The listing builds one solid part. Answer for the finished solid, in the listing's coordinates (mm). Face numbers are marked on the shaded views. A direction names the side the tool comes from. Round coordinates to 2 decimals unless told otherwise and drop trailing zeros. Write each loop counter-clockwise with the first axis right and the second up, starting at its lowest first coordinate (ties: lowest second). Pieces come first, ordered by that corner, then holes. Notation, with made-up numbers: M -33,26.5 L 10,26.5 A21 cw 10,35.5 Z; hole C 34,77 d1. An arc over 180 degrees is marked long. Write each question's results on one line, items separated by ' | '.
from build123d import *

# Parameters (mm, degrees)
CROQUIS1_W              = 50
CROQUIS1_H              = 100
SALIENTE_EXTRUIR1_DEPTH = 6
CROQUIS2_W              = 50
CROQUIS2_H              = 6
SALIENTE_EXTRUIR2_DEPTH = 276
CROQUIS3_R              = 13
CORTAR_EXTRUIR1_DEPTH   = 6
REDONDEO1_R             = 20


with BuildPart() as part:
    # Croquis1 → Saliente-Extruir1 (new body)
    with BuildSketch(Plane(origin=(0, 0, 0), x_dir=(1, 0, 0), z_dir=(0, 1, 0))):
        Rectangle(CROQUIS1_W, CROQUIS1_H)
    extrude(amount=SALIENTE_EXTRUIR1_DEPTH)

    # Croquis2 → Saliente-Extruir2 (add)
    with BuildSketch(Plane.XZ):
        with Locations((0, 53)):
            Rectangle(CROQUIS2_W, CROQUIS2_H)
    extrude(amount=-SALIENTE_EXTRUIR2_DEPTH)

    # Croquis3 → Cortar-Extruir1 (cut)
    with BuildSketch(Plane.XY.offset(56)):
        with Locations((0, 246)):
            Circle(CROQUIS3_R)
    extrude(amount=-CORTAR_EXTRUIR1_DEPTH, mode=Mode.SUBTRACT)

    # Redondeo1
    redondeo1_edges = [part.edges().sort_by_distance(p)[0] for p in [
        (25, 276, 53),
        (-25, 276, 53),
    ]]
    fillet(redondeo1_edges, radius=REDONDEO1_R)


solid = part.part
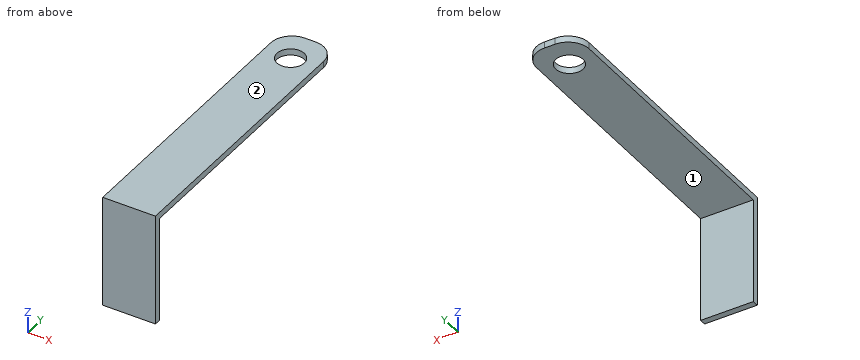
1) Find the intervals of material crossed by line 1 (Y direction, x = 0, z = 51.4); line 2 (Z direction, x = 11, y = 161); line 3 (Y direction, x = -17.5, z = -36), in increasing order.
Return value:
line 1: 0 to 233, 259 to 276 | line 2: 50 to 56 | line 3: 0 to 6
2) Section C-C (z = 11) is taken. Determine the outline of the cut face in (x, y).
Return value:
outline: M -25,0 L 25,0 L 25,6 L -25,6 Z
3) A tool of negligible diameter and unlimited length cuts with its end or side. For the marked faces 1 and 2, from which of +Z, -Z, +X, -X, +Y, -Y can it reach the whole face along a straight path? Write none if from no direction.
Return value:
face 1: -Z, +X, -X, +Y | face 2: +Z, +X, -X, +Y, -Y
4) Each of these flat-tipped pins is pushed along its axis until it touches: pin 1 (10 mm diameter, centred on x = -18.5, z = 31, fed in from +Y); pin 2 (25 mm diameter, centred on x = 8.5, y = 131, fed in from -Z). Where does it stop, or does it pass through?
Return value:
pin 1: y = 6 | pin 2: z = 50
5) Section A-A (y = 246) is taken. Determine the outline of the cut face in (x, z), then the cut area to 3 significant figures.
Return value:
outline: M -25,50 L -13,50 L -13,56 L -25,56 Z; M 13,50 L 25,50 L 25,56 L 13,56 Z | area: 144 mm²
6) Section B-B (x = 0) is taken. Determine the outline of the cut face in (y, z), then the cut area to 3 significant figures.
Return value:
outline: M 0,-50 L 6,-50 L 6,50 L 233,50 L 233,56 L 0,56 Z; M 259,50 L 276,50 L 276,56 L 259,56 Z | area: 2,100 mm²
7) Section D-D (x = 20) is taken. Determine the outline of the cut face in (y, z).
Return value:
outline: M 0,-50 L 6,-50 L 6,50 L 269.23,50 L 269.23,56 L 0,56 Z
